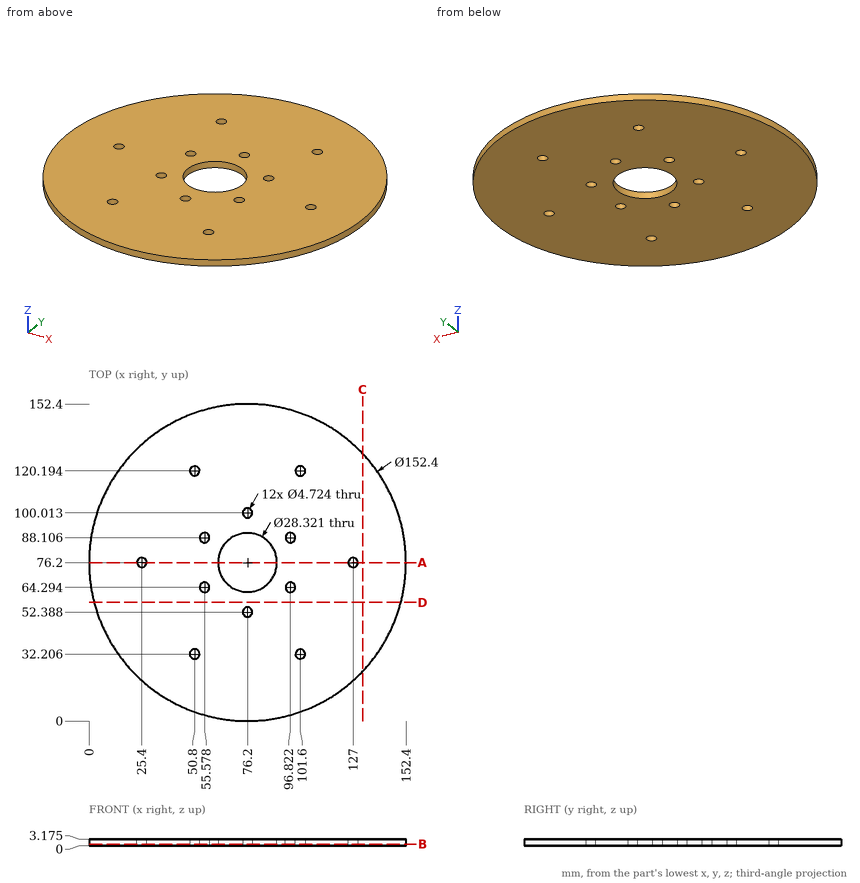
Part print with two shaded views. Sizes in mm from the minimum x, y, z corner. Coordinates: 2 decimals unless noted, no trailing zeros. Order: outer loops, then holes, each group sorted by start corner. A loop starts at its lowest first (then second) coordinate and runs counter-clockwise, first axis right, second up. Notation, with made-up numbers: (19, -25.5) - (31, -25.5) arc R16 cw to (31, -6.5) - close; hole circle Ø10 at (41, -17.5). An arc over 180 degrees is marked (long way). Write item = value, one per line. Start each with the question number.
1) Saw through at D-D on y = 57. Write the cut outline in (x, z) (1 decimal).
2) Flat gauge pins, fed straight in: pin 1 Ø3 at (x, y) = (96.82, 64.29) entering from -Z; pin 2 Ø6 at (x, y) = (55.58, 88.11) entering from -Z. Where does each tip first touch, or does it go through?
3) Saw through at C-C on x = 131.5. Write the cut outline in (y, z) (1 decimal).
4) Saw through at B-B on z = 0.75. Count the separate pieces of the cut face and the enclosed holes in it, then the cut area to 3 significant figures.
5) Wall check: line 1 along Y through (x, z) = (50.8, 1.4) (1 decimal); line 2 along X through (y, z) = (121.5, 2) (1 decimal); line 3 along X through (y, z) = (30.5, 2.6) (1 decimal). Give the ranges that are in metal, low to high. Write a range as from..to.
6) Saw through at A-A on y = 76.2. Write the cut outline in (x, z) (1 decimal), then the cut area to 3 significant figures.
From the geometry:
q1.outline = (2.5, 0) - (149.9, 0) - (149.9, 3.2) - (2.5, 3.2) - close
q2.pin_1 = through
q2.pin_2 = 0
q3.outline = (23.8, 0) - (128.6, 0) - (128.6, 3.2) - (23.8, 3.2) - close
q4.separate_pieces = 1
q4.enclosed_holes = 13
q4.area = 17,400 mm^2
q5.line_1 = 4.4..29.8, 34.6..117.8, 122.6..148
q5.line_2 = 14.9..48.8, 52.8..99.6, 103.6..137.5
q5.line_3 = 15.2..49.2, 52.4..100, 103.2..137.2
q6.outline = (0, 0) - (23, 0) - (23, 3.2) - (0, 3.2) - close; (27.8, 0) - (62, 0) - (62, 3.2) - (27.8, 3.2) - close; (90.4, 0) - (124.6, 0) - (124.6, 3.2) - (90.4, 3.2) - close; (129.4, 0) - (152.4, 0) - (152.4, 3.2) - (129.4, 3.2) - close
q6.area = 364 mm^2
